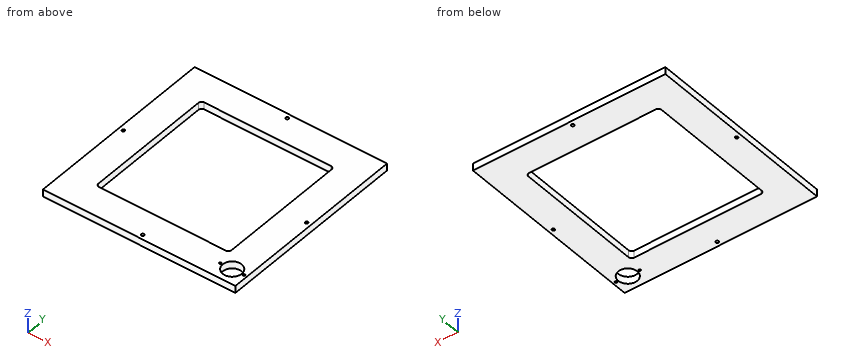
from build123d import *

# Parameters (mm, degrees)
SKETCH_W        = 324
SKETCH_H        = 324
PAD_DEPTH       = 12
POCKET_DEPTH    = 12.001
SKETCH002_R     = 2.5
POCKET001_DEPTH = 12.001
SKETCH003_R     = 16
SKETCH003_R_2   = 1.75
POCKET002_DEPTH = 12.001


with BuildPart() as part:
    # Sketch → Pad (new body)
    with BuildSketch(Plane.XY):
        Rectangle(SKETCH_W, SKETCH_H)
    extrude(amount=PAD_DEPTH)

    # Sketch001 (on Face6 of Pad) → Pocket (cut, through all)
    with BuildSketch(Plane.XY.offset(12)):
        with BuildLine():
            Line((-112, 107.000007), (-112, -106.999984))
            ThreePointArc((-112, -106.999984), (-110.535541, -110.535527), (-107.000004, -112))
            Line((-107.000004, -112), (107.000004, -112))
            ThreePointArc((107.000004, -112), (110.535542, -110.535526), (112, -106.999982))
            Line((112, 107.000009), (112, -106.999982))
            ThreePointArc((112, 107.000009), (110.535532, 110.535536), (107.000003, 112))
            Line((-107.000005, 112), (107.000003, 112))
            ThreePointArc((-107.000005, 112), (-110.535533, 110.535535), (-112, 107.000007))
        make_face()
    extrude(amount=-POCKET_DEPTH, mode=Mode.SUBTRACT)

    # Sketch002 (on Face5 of Pocket) → Pocket001 (cut, through all)
    with BuildSketch(Plane.XY.offset(12)):
        with Locations((0, 154.5)):
            Circle(SKETCH002_R)
        with Locations((-154.5, 0)):
            Circle(SKETCH002_R)
        with Locations((154.5, 0)):
            Circle(SKETCH002_R)
        with Locations((0, -154.5)):
            Circle(SKETCH002_R)
    extrude(amount=-POCKET001_DEPTH, mode=Mode.SUBTRACT)

    # Sketch003 (on Face5 of Pocket001) → Pocket002 (cut, through all)
    with BuildSketch(Plane.XY.offset(12)):
        with Locations((137, -137)):
            Circle(SKETCH003_R)
        with Locations((117.1, -137)):
            Circle(SKETCH003_R_2)
        with Locations((156.9, -137)):
            Circle(SKETCH003_R_2)
    extrude(amount=-POCKET002_DEPTH, mode=Mode.SUBTRACT)


solid = part.part
Geometry: final body of the model. Coordinates: model frame, mm. Coordinates: 2 decimals unless noted, no trailing zeros. Loops run counter-clockwise (first coordinate to the right, second up) from the corner with the lowest first, then second, coordinate; pieces in that order, holes last. Notation, with made-up numbers: (-10, 29) - (42, 29) arc R21 cw to (42, 66) - close; hole circle Ø4 at (24.5, 34). An arc over 180 degrees is marked (long way). Put each result on its own line as item: value. Start each with the question number.
Q1. Pin query (flat end, axial travel): pin 1 Ø4.5 at (x, y) = (156.9, -137) entering from +Z. Return the tip coordinate at first contact, or that it passes through.
Q2. Line query: line 1 (Y direction, x = 0, z = 5); line 2 (Y direction, x = 89, z = 2.25); line 3 (X direction, y = -154.5, z = 6.5). Output: solid intervals per line, ascending.
Q3. Cut plane A-A, the plane x = -39.5. Return loops of the section in (y, z), and give its area (3 significant figures).
Q4. Cut plane C-C, the plane z = 6. Give the number of separate pieces and of enclosed holes in the cut face, and give its area (3 significant figures).
Filled sheet:
1. pin 1: z = 12
2. line 1: -162 to -157, -152 to -112, 112 to 152, 157 to 162
2. line 2: -162 to -112, 112 to 162
2. line 3: -162 to -2.5, 2.5 to 162
3. outline: (-162, 0) - (-112, 0) - (-112, 12) - (-162, 12) - close; (112, 0) - (162, 0) - (162, 12) - (112, 12) - close
3. area: 1,200 mm²
4. separate pieces: 1
4. enclosed holes: 8
4. area: 53,900 mm²
